from build123d import *

# Parameters (mm, degrees)
CROQUIS1_W              = 81
CROQUIS1_H              = 47
SALIENTE_EXTRUIR1_DEPTH = 3
CORTAR_EXTRUIR2_DEPTH   = 47.920144927
CROQUIS2_R              = 1.6
CORTAR_EXTRUIR1_DEPTH   = 47.920144927
CROQUIS5_R              = 1
CROQUIS5_W              = 16
CROQUIS5_H              = 59.242740908
CROQUIS5_W_2            = 21.5
CROQUIS5_H_2            = 2.5
CORTAR_EXTRUIR4_DEPTH   = 10
CORTAR_EXTRUIR5_DEPTH   = 10
CROQUIS7_W              = 27.893037997
CROQUIS7_H              = 58.785327392
CORTAR_EXTRUIR6_DEPTH   = 10
CROQUIS8_W              = 8
CROQUIS8_H              = 24
CROQUIS8_R              = 1.6
SALIENTE_EXTRUIR2_DEPTH = 3
REDONDEO1_R             = 4
REDONDEO4_R             = 5
REDONDEO3_SIZE          = 4


# Some blends are built 0.0001 mm under size
with BuildPart() as part:
    # Croquis1 → Saliente-Extruir1 (new body)
    with BuildSketch(Plane(origin=(0, 0, 0), x_dir=(1, 0, 0), z_dir=(0, 1, 0))):
        Rectangle(CROQUIS1_W, CROQUIS1_H)
    extrude(amount=SALIENTE_EXTRUIR1_DEPTH)

    # Croquis3 → Cortar-Extruir2 (cut, through all)
    with BuildSketch(Plane(origin=(0, 3, 0), x_dir=(1, 0, 0), z_dir=(0, 1, 0))):
        Polygon((-32.5, 23.5), (23.5, 23.5), (23.5, 13.5), (-4.5, 13.5), (-4.5, 5), (-32.5, 5), align=None)
        Polygon((-32.5, -5), (-32.5, -23.5), (23.5, -23.5), (23.5, -13.5), (-4.5, -13.5), (-4.5, -5), align=None)
    extrude(amount=-CORTAR_EXTRUIR2_DEPTH, mode=Mode.SUBTRACT)

    # Croquis2 → Cortar-Extruir1 (cut, through all)
    with BuildSketch(Plane(origin=(0, 3, 0), x_dir=(1, 0, 0), z_dir=(0, 1, 0))):
        with Locations(Location((-36.5, 19.5, 0), (0, 0, 270))):
            Circle(CROQUIS2_R)
        with Locations(Location((-36.5, -19.5, 0), (0, 0, 270))):
            Circle(CROQUIS2_R)
        with Locations(Location((27.5, 19.5, 0), (0, 0, 270))):
            Circle(CROQUIS2_R)
        with Locations(Location((27.5, -19.5, 0), (0, 0, 270))):
            Circle(CROQUIS2_R)
        with Locations(Location((-36.5, 11.5, 0), (0, 0, 270))):
            Circle(CROQUIS2_R)
        with Locations(Location((-36.5, -11.5, 0), (0, 0, 270))):
            Circle(CROQUIS2_R)
    extrude(amount=-CORTAR_EXTRUIR1_DEPTH, mode=Mode.SUBTRACT)

    # Croquis5 → Cortar-Extruir4 (cut)
    with BuildSketch(Plane(origin=(0, 3, 0), x_dir=(1, 0, 0), z_dir=(0, 1, 0))):
        with Locations(Location((-0.6, 6.18, 0), (0, 0, 270))):
            Circle(CROQUIS5_R)
        with Locations(Location((31, 8.82, 0), (0, 0, 270))):
            Circle(CROQUIS5_R)
        with Locations(Location((31, -8.82, 0), (0, 0, 270))):
            Circle(CROQUIS5_R)
        with Locations(Location((-0.6, -6.82, 0), (0, 0, 270))):
            Circle(CROQUIS5_R)
        with Locations((42.5, 1.68576905)):
            Rectangle(CROQUIS5_W, CROQUIS5_H)
        with Locations((11.65, 10.25)):
            Rectangle(CROQUIS5_W_2, CROQUIS5_H_2)
    extrude(amount=-CORTAR_EXTRUIR4_DEPTH, mode=Mode.SUBTRACT)

    # Croquis6 → Cortar-Extruir5 (cut)
    with BuildSketch(Plane(origin=(0, 3, 0), x_dir=(1, 0, 0), z_dir=(0, 1, 0))):
        with BuildLine():
            Line((-19.5, 1.6), (-15.5, 1.6))
            ThreePointArc((-15.5, 1.6), (-13.9, 0), (-15.5, -1.6))
            Line((-15.5, -1.6), (-19.5, -1.6))
            ThreePointArc((-19.5, -1.6), (-21.1, 0), (-19.5, 1.6))
        make_face()
    extrude(amount=-CORTAR_EXTRUIR5_DEPTH, mode=Mode.SUBTRACT)

    # Croquis7 → Cortar-Extruir6 (cut)
    with BuildSketch(Plane(origin=(0, 3, 0), x_dir=(1, 0, 0), z_dir=(0, 1, 0))):
        with Locations((-38.446518998, -0.587422332)):
            Rectangle(CROQUIS7_W, CROQUIS7_H)
    extrude(amount=-CORTAR_EXTRUIR6_DEPTH, mode=Mode.SUBTRACT)

    # Croquis8 → Saliente-Extruir2 (add, through all)
    with BuildSketch(Plane(origin=(0, 3, 0), x_dir=(1, 0, 0), z_dir=(0, 1, 0))):
        with Locations((20.5, -25.5)):
            Rectangle(CROQUIS8_W, CROQUIS8_H)
        with Locations(Location((20.5, -33.5, 0), (0, 0, 270))):
            Circle(CROQUIS8_R, mode=Mode.SUBTRACT)
    saliente_extruir2 = extrude(amount=-SALIENTE_EXTRUIR2_DEPTH)

    # Simetría1: Saliente-Extruir2 across plane
    add(saliente_extruir2.mirror(Plane.XY))

    # Redondeo1
    redondeo1_edges = [part.edges().sort_by_distance(p)[0] for p in [
        (34.5, 1.5, 23.5),
        (34.5, 1.5, -23.5),
        (16.5, 1.5, 37.5),
        (24.5, 1.5, 37.5),
        (16.5, 1.5, 13.5),
        (24.5, 1.5, 23.5),
        (24.5, 1.5, -37.5),
        (16.5, 1.5, -37.5),
        (16.5, 1.5, -13.5),
        (24.5, 1.5, -23.5),
    ]]
    fillet(redondeo1_edges, radius=REDONDEO1_R - 0.0001)  # a hair under: the kernel refuses the full size

    # Redondeo4
    redondeo4_edges = [part.edges().sort_by_distance(p)[0] for p in [
        (-24.5, 1.5, -5),
        (-24.5, 1.5, 5),
    ]]
    fillet(redondeo4_edges, radius=REDONDEO4_R - 0.0001)  # a hair under: the kernel refuses the full size

    # Redondeo3
    # a fillet whose section is not a circle: 4 mm, written as the material it adds along each edge
    with BuildSketch(Plane(origin=(-4.5, 3, 5), x_dir=(-1, 0, 0), z_dir=(0, -1, 0))) as redondeo3_piece_1:
        with BuildLine():
            Bezier((REDONDEO3_SIZE, 0), (0, 0), (0, -REDONDEO3_SIZE), weights=[1, 1.5, 1])
            Line((0, -REDONDEO3_SIZE), (0, 0))
            Line((0, 0), (REDONDEO3_SIZE, 0))
        make_face()
    extrude(amount=3)
    with BuildSketch(Plane(origin=(-4.5, 3, -5), x_dir=(-1, 0, 0), z_dir=(0, -1, 0))) as redondeo3_piece_2:
        with BuildLine():
            Bezier((REDONDEO3_SIZE, 0), (0, 0), (0, REDONDEO3_SIZE), weights=[1, 1.5, 1])
            Line((0, REDONDEO3_SIZE), (0, 0))
            Line((0, 0), (REDONDEO3_SIZE, 0))
        make_face()
    extrude(amount=3)
    # a fillet whose section is not a circle: 4 mm, written as the material it takes off along each edge
    with BuildSketch(Plane(origin=(-4.5, 13, 13.5), x_dir=(0, 0, -1), z_dir=(0, -1, 0))) as redondeo3_2_piece_1:
        with BuildLine():
            Bezier((REDONDEO3_SIZE, 0), (0, 0), (0, REDONDEO3_SIZE), weights=[1, 1.5, 1])
            Line((0, REDONDEO3_SIZE), (0, 0))
            Line((0, 0), (REDONDEO3_SIZE, 0))
        make_face()
    extrude(amount=23, mode=Mode.SUBTRACT)
    with BuildSketch(Plane(origin=(-4.5, 13, -13.5), x_dir=(0, 0, 1), z_dir=(0, -1, 0))) as redondeo3_2_piece_2:
        with BuildLine():
            Bezier((REDONDEO3_SIZE, 0), (0, 0), (0, -REDONDEO3_SIZE), weights=[1, 1.5, 1])
            Line((0, -REDONDEO3_SIZE), (0, 0))
            Line((0, 0), (REDONDEO3_SIZE, 0))
        make_face()
    extrude(amount=23, mode=Mode.SUBTRACT)


solid = part.part
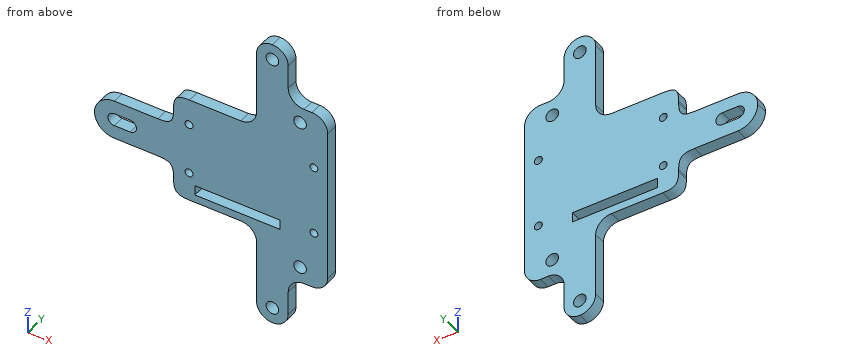
Design review of the part built by this model. Coordinates are the model's own, in mm. Coordinates: 2 decimals unless noted, no trailing zeros. Loops run counter-clockwise (first coordinate to the right, second up) from the corner with the lowest first, then second, coordinate; pieces in that order, holes last.
Item 1: Clearance check with flat-ended pins moving along their axes: pin 1 (1.8 mm diameter, centred on x = 31, z = -8.82, fed in from +Y); pin 2 (1.5 mm diameter, centred on y = 1.5, z = 29, fed in from +X); pin 3 (0.6 mm diameter, centred on y = 1, z = -9.5, fed in from -X); pin 4 (0.9 mm diameter, centred on x = 12, y = 1.5, fed in from +Z). State where each tip first meets the part, or that it passes through.
Completed:
pin 1: passes through
pin 2: stops at x = 24.5
pin 3: stops at x = -4.5
pin 4: stops at z = 13.5
Item 2: Wall thickness on L1, parallel to X at y = 2.3, z = 9; L2, parallel to Z at x = 27, y = 0.75; L3, parallel to X at y = 1.85, z = -33.5: over which ranges is each line inside the solid? List them lowest first.
Completed:
L1: x = -4.5 to 30.02, 31.98 to 34.5
L2: z = -23.79 to -21.02, -17.98 to 17.98, 21.02 to 23.79
L3: x = 16.5 to 18.9, 22.1 to 24.5
Item 3: Add section C-C (z = -30). Write out the cut boundary in (x, y).
Completed:
outline: (16.5, 0) - (24.5, 0) - (24.5, 3) - (16.5, 3) - close
Item 4: Add section A-A (x = 27.5). Write out the cut boundary in (y, z).
Completed:
outline: (0, -23.63) - (3, -23.63) - (3, -21.1) - (0, -21.1) - close; (0, -17.9) - (3, -17.9) - (3, 17.9) - (0, 17.9) - close; (0, 21.1) - (3, 21.1) - (3, 23.63) - (0, 23.63) - close
Item 5: Add section B-B (y = 0.7). Give the number of separate pieces and of enclosed holes in the cut face, and give its area (3 significant figures).
Completed:
separate pieces: 1
enclosed holes: 10
area: 1,700 mm2
